Geometry: final body of the model. Coordinates: model frame, mm. A direction names the side the tool comes from. Round coordinates to 2 decimals unless told otherwise and drop trailing zeros. Write each loop counter-clockwise with the first axis right and the second up, starting at its lowest first coordinate (ties: lowest second). Pieces come first, ordered by that corner, then holes. Notation, with made-up numbers: (33.5, -23) -> (45.5, -23) arc R26 cw to (45.5, -6) -> close; hole circle Ø10 at (81.25, 81.5). An arc over 180 degrees is marked (long way). Use one line per item in the form item = value. Start each with the question number.
1. Draft query along Y for faces 6 (the face through (905, 435.5, -7)), 7 (the face through (905, 18.3, 1)), 8 (the face through (905, -2, 18.148)), 9 (the face through (913, 3, 21.148)). Return one class per face: pulls with the +Y half, pulls with the -Y half, needs draft (parallel to the pull), parting line crosses it, or undercut.
2. Reachability of faces 1 (the face through (905, -2, -18.852)), 2 (the face through (905, -21.7, -7)), 3 (the face through (905, -2, -15.852)), 4 (the face through (1834.8, 204, -28)), 5 (the face through (1828.8, 204, -28)) from +Z, -Z, +X, -X, +Y, -Y: full face, straight path, thin tool, end or side. Return the list, or none.
3. Pin query (flat end, axial travel): pin 1 Ø17 at (x, y) = (1254, 418.5) entering from -Z. Return the tip coordinate at first contact, or that it passes through.
4. Cut plane C-C, the plane z = -63. Return the cut outline in (x, y), plus the area to 3 significant figures.
5. Cut plane B-B, the plane y = 364. Return the cut outline in (x, z).
6. Cut plane A-A, the plane x = 1148.5. Return the cut outline in (y, z), plus the area to 3 significant figures.
7. Line query: L1, parallel to Y at x = 1630, z = -7; L2, parallel to X at y = 67, z = 11.5; L3, parallel to Z at x = 463, y = 9. Output: solid intervals per line, ascending.
```python
from build123d import *

# Parameters (mm, degrees)
F0_W     = 40
F0_H     = 40
F0_W_2   = 34
F0_H_2   = 34
F1_DEPTH = 1828.8
F2_W     = 457.2
F2_H     = 100
F3_DEPTH = 6
F4_W     = 40
F4_H     = 40
F4_W_2   = 34
F4_H_2   = 34
F5_DEPTH = 1828.8
F6_W     = 457.2
F6_H     = 100
F7_DEPTH = 6


with BuildPart() as f1:
    # F0 (on Right) → F1 (new body)
    with BuildSketch(Plane.YZ):
        with Locations((-1.69964, 1.148437)):
            Rectangle(F0_W, F0_H)
        with Locations((-1.69964, 1.148437)):
            Rectangle(F0_W_2, F0_H_2, mode=Mode.SUBTRACT)
    extrude(amount=F1_DEPTH)

    # F2 (on Right) → F3 (join)
    with BuildSketch(Plane.YZ):
        with Locations((206.90036, -28.851563)):
            Rectangle(F2_W, F2_H)
    extrude(amount=F3_DEPTH)

    # F4 (on face) → F5 (join)
    with BuildSketch(Plane.YZ.offset(6)):
        with Locations((415.50036, 1.148437)):
            Rectangle(F4_W, F4_H)
        with Locations((415.50036, 1.148437)):
            Rectangle(F4_W_2, F4_H_2, mode=Mode.SUBTRACT)
    extrude(amount=F5_DEPTH)

    # F6 (on face) → F7 (join)
    with BuildSketch(Plane.YZ.offset(1828.8)):
        with Locations((206.90036, -28.851563)):
            Rectangle(F6_W, F6_H)
    extrude(amount=F7_DEPTH)


solid = f1.part
```
Outcome:
q1.face_6 = pulls with the +Y half
q1.face_7 = undercut
q1.face_8 = undercut
q1.face_9 = needs draft
q2.face_1 = -Z, +Y, -Y
q2.face_2 = +Z, -Z, +X, -X, -Y
q2.face_3 = none
q2.face_4 = +Z, -Z, +X, +Y, -Y
q2.face_5 = -Z
q3.pin_1 = -18.85
q4.outline = (0, -21.7) -> (6, -21.7) -> (6, 435.5) -> (0, 435.5) -> close; (1828.8, -21.7) -> (1834.8, -21.7) -> (1834.8, 435.5) -> (1828.8, 435.5) -> close
q4.area = 5,490 mm^2
q5.outline = (0, -78.85) -> (6, -78.85) -> (6, 21.15) -> (0, 21.15) -> close; (1828.8, -78.85) -> (1834.8, -78.85) -> (1834.8, 21.15) -> (1828.8, 21.15) -> close
q6.outline = (-21.7, -18.85) -> (18.3, -18.85) -> (18.3, 21.15) -> (-21.7, 21.15) -> close; (395.5, -18.85) -> (435.5, -18.85) -> (435.5, 21.15) -> (395.5, 21.15) -> close; hole (-18.7, -15.85) -> (15.3, -15.85) -> (15.3, 18.15) -> (-18.7, 18.15) -> close; hole (398.5, -15.85) -> (432.5, -15.85) -> (432.5, 18.15) -> (398.5, 18.15) -> close
q6.area = 888 mm^2
q7.L1 = -21.7 to -18.7, 15.3 to 18.3, 395.5 to 398.5, 432.5 to 435.5
q7.L2 = 0 to 6, 1828.8 to 1834.8
q7.L3 = -18.85 to -15.85, 18.15 to 21.15
